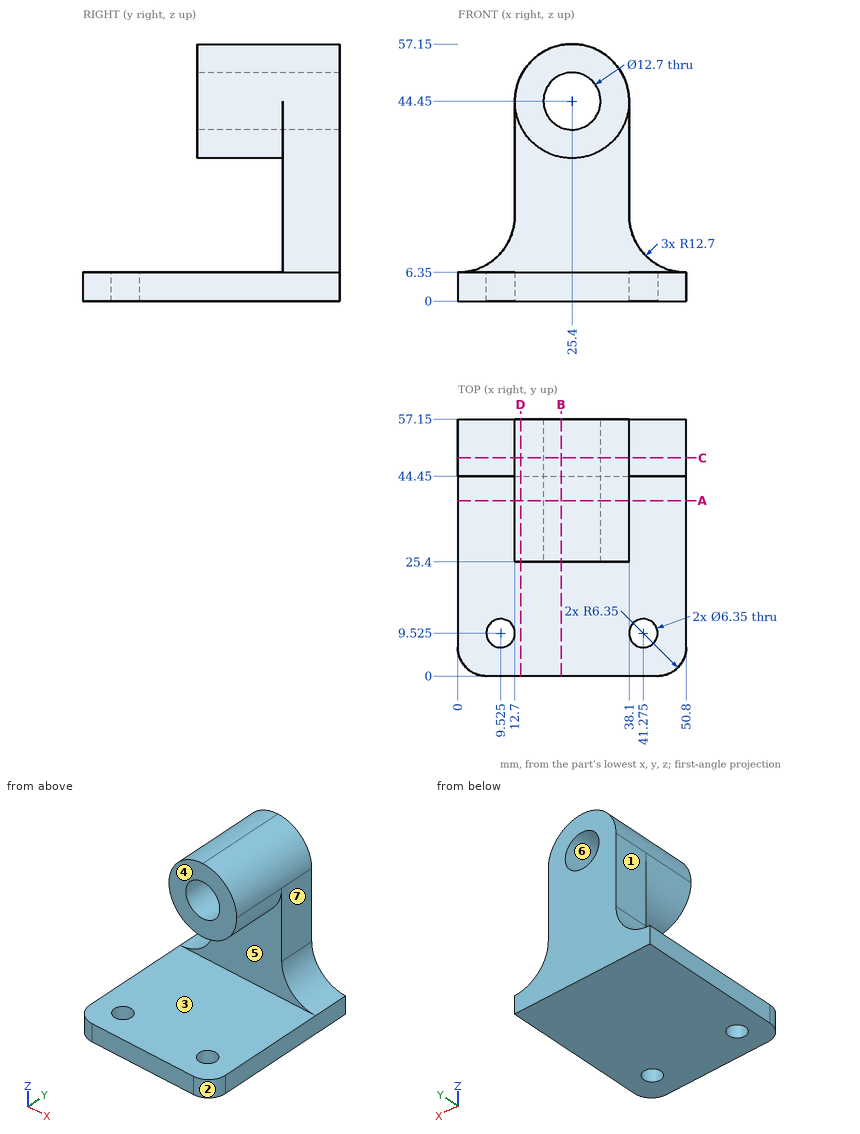
The figure shows three views and two pictorial views of one solid part (mm, origin at its lowest corner). Answer the questions. A direction names the side the tool comes from. Give positions to 0.01 mm unless a question says otherwise; leave off trailing zeros. Order: outer loops, then holes, each group sorted by start corner. A loop starts at its lowest first (then second) coordinate and runs counter-clockwise, first axis right, second up. Notation, with made-up numbers: (62.25, 66.5) -> (117.25, 66.5) arc R21 cw to (117.25, 77.5) -> close; hole circle Ø8 at (13.5, -5). An arc over 180 degrees is marked (long way). Write each question's results on one line, items separated by ' | '.
Q1. Each of these flat-tipped pins is pushed along its axis until it touches: P1, Ø14, axis at y = 47.5, z = 35, coming from the +X side; P2, Ø7.5, axis at x = 25.4, z = 44.45, coming from the +Y side; P3, Ø1, axis at y = 44.5, z = 15, coming from the +X side; P4, Ø12.5, axis at x = 20.5, z = 49.5, coming from the -Y side. Where does it stop, or does it pass through?
Checked values:
P1: stops at x = 38.1 | P2: passes through | P3: stops at x = 38.94 | P4: stops at y = 25.4
Q2. Straight lines are drawn through the part: probe 1 along Z at (x, y) = (25, 26.5); probe 2 along Z at (x, y) = (26.5, 33.5); probe 3 along Y at (x, z) = (35.5, 49). For each, find the intervals that lie inside material, in ascending order. Write a range as from..to.
Checked values:
probe 1: z = 0..6.35, 31.76..38.11, 50.79..57.14 | probe 2: z = 0..6.35, 31.8..38.2, 50.7..57.1 | probe 3: y = 25.4..57.15
Q3. Which of the six approach directions +Z, -Z, +X, -X, +Y, -Y give full straight-line access (tool end or side, diameter ignored) to the marked faces 1, 2, 3 and 4?
Checked values:
face 1: +Z, -X, +Y, -Y | face 2: +Z, -Z, +X, -Y | face 3: +X, -X, -Y | face 4: +Z, +X, -X, -Y
Q4. The part is cut by section C-C, the plane y = 48.5. Give the vertices of the cut face in (x, z).
Checked values:
outline: (0, 0) -> (50.8, 0) -> (50.8, 6.35) arc R12.7 cw to (38.1, 19.05) -> (38.1, 44.45) arc R12.7 ccw to (12.7, 44.45) -> (12.7, 19.05) arc R12.7 cw to (0, 6.35) -> close; hole circle Ø12.7 at (25.4, 44.45)
Q5. The part is cut by section A-A, the plane y = 39. Give the vertices of the cut face in (x, z).
Checked values:
outline: (0, 0) -> (50.8, 0) -> (50.8, 6.35) -> (0, 6.35) -> close; circle Ø25.4 at (25.4, 44.45); hole circle Ø12.7 at (25.4, 44.45)
Q6. Determine the mould class of the marked faces 5, 6 and 7 for opening direction X: pulls with the +X half, pulls with the -X half, needs draft (parallel to the pull), parting line crosses it, or undercut.
Checked values:
face 5: needs draft | face 6: undercut | face 7: pulls with the +X half
Q7. The part is cut by section B-B, the plane x = 23. Give the vertices of the cut face in (y, z), and give its area (3 significant figures).
Checked values:
outline: (0, 0) -> (57.15, 0) -> (57.15, 38.57) -> (25.4, 38.57) -> (25.4, 31.98) -> (44.45, 31.98) -> (44.45, 6.35) -> (0, 6.35) -> close; (25.4, 50.33) -> (57.15, 50.33) -> (57.15, 56.92) -> (25.4, 56.92) -> close | area: 1,110 mm^2
Q8. The part is cut by section D-D, the plane x = 14. Give the vertices of the cut face in (y, z), and give its area (3 significant figures).
Checked values:
outline: (0, 0) -> (57.15, 0) -> (57.15, 50.05) -> (25.4, 50.05) -> (25.4, 38.85) -> (44.45, 38.85) -> (44.45, 6.35) -> (0, 6.35) -> close | area: 1,130 mm^2
